Input: part model. Units: mm. Frame: model coordinates. A direction names the side the tool comes from. Round coordinates to 2 decimals unless told otherwise and drop trailing zeros. Loops run counter-clockwise (first coordinate to the right, second up) from the corner with the lowest first, then second, coordinate; pieces in that order, holes last. Notation, with made-up numbers: (0, -13) -> (35, -13) arc R25 ccw to (35, 14) -> close; hole circle Ø9 at (-5.5, 52). An arc over 180 degrees is marked (long way). Answer as a JSON object with one key per item and string values.
```python
from build123d import *

# Parameters (mm, degrees)
F0_W      = 12.7
F0_H      = 12.7
F1_DEPTH  = 76.2
F2_W      = 12.7
F2_H      = 25.4
F3_DEPTH  = 9.525
F4_W      = 12.7
F4_H      = 25.4
F5_DEPTH  = 9.525
F7_DEPTH  = 9.525
F9_DEPTH  = 9.525
F10_R     = 3.1496
F11_DEPTH = 25.4
F12_R     = 3.1496
F13_DEPTH = 25.4
F14_SIZE  = 2.54


with BuildPart() as f1:
    # F0 (on Top) → F1 (new body, symmetric)
    with BuildSketch(Plane.XY):
        Rectangle(F0_W, F0_H)
    extrude(amount=F1_DEPTH, both=True)

    # F2 (on face) → F3 (join)
    with BuildSketch(Plane(origin=(0, 6.35, 0), x_dir=(-1, 0, 0), z_dir=(0, 1, 0))):
        with Locations((0, -58.42)):
            Rectangle(F2_W, F2_H)
        with Locations((0, -12.7)):
            Rectangle(F2_W, F2_H)
        with Locations((0, 33.02)):
            Rectangle(F2_W, F2_H)
    extrude(amount=F3_DEPTH)

    # F4 (on face) → F5 (join)
    with BuildSketch(Plane.XZ.offset(6.35)):
        with Locations((0, 48.26)):
            Rectangle(F4_W, F4_H)
        with Locations((0, 2.54)):
            Rectangle(F4_W, F4_H)
        with Locations((0, -43.18)):
            Rectangle(F4_W, F4_H)
    extrude(amount=F5_DEPTH)

    # F6 (on face) → F7 (join)
    with BuildSketch(Plane(origin=(-6.35, 0, 0), x_dir=(0, -1, 0), z_dir=(-1, 0, 0))):
        Polygon((-6.35, 66.260369), (-6.35, 45.72), (-6.35, 44.788861), (6.35, 44.788861), (6.35, 60.96), (6.35, 66.260369), align=None)
        Polygon((-6.35, 20.32), (-6.35, 0), (6.35, 0), (6.35, 15.24), (6.35, 22.712743), (-6.35, 22.712743), align=None)
        Polygon((-6.35, -45.72), (-6.35, -50.8), (0, -50.8), (0, -19.05), (-6.35, -19.05), (-6.35, -25.4), align=None)
    extrude(amount=F7_DEPTH)

    # F8 (on face) → F9 (join)
    with BuildSketch(Plane.YZ.offset(6.35)):
        Polygon((6.35, -24.37056), (-6.35, -24.37056), (-6.35, -30.48), (-6.35, -49.77056), (6.35, -49.77056), (6.35, -45.72), (6.35, -25.4), align=None)
        Polygon((6.35, 35.56), (-6.35, 35.56), (-6.35, 15.24), (-6.35, 10.16), (6.35, 10.16), (6.35, 20.32), align=None)
        Polygon((6.35, 73.66), (-6.35, 73.66), (-6.35, 60.96), (-6.35, 48.26), (6.35, 48.26), align=None)
    extrude(amount=F9_DEPTH)

    # F10 (on face) → F11 (join)
    with BuildSketch(Plane.XY.offset(76.2)):
        Circle(F10_R)
    extrude(amount=F11_DEPTH)

    # F12 (on face) → F13 (join)
    with BuildSketch(Plane(origin=(0, 0, -76.2), x_dir=(1, 0, 0), z_dir=(0, 0, -1))):
        Circle(F12_R)
    extrude(amount=F13_DEPTH)

    # F14
    f14_edges = [f1.edges().sort_by_distance(p)[0] for p in [
        (15.875, -6.35, 60.96),
        (15.875, 6.35, 60.96),
        (6.35, -15.875, 48.26),
        (-6.35, -15.875, 48.26),
        (-15.875, -6.35, 55.524615),
        (-15.875, 6.35, 55.524615),
        (-6.35, 15.875, 33.02),
        (6.35, 15.875, 33.02),
        (15.875, 6.35, 22.86),
        (15.875, -6.35, 22.86),
        (6.35, -15.875, 2.54),
        (-6.35, -15.875, 2.54),
        (-15.875, -6.35, 11.356371),
        (-15.875, 6.35, 11.356371),
        (-6.35, 15.875, -12.7),
        (6.35, 15.875, -12.7),
        (-15.875, 6.35, -34.925),
        (-15.875, 0, -34.925),
        (-6.35, -15.875, -43.18),
        (6.35, -15.875, -43.18),
        (6.35, -6.35, -40.12528),
        (15.875, 6.35, -37.07056),
        (15.875, -6.35, -37.07056),
        (6.35, 15.875, -58.42),
        (-6.35, 15.875, -58.42),
    ]]
    chamfer(f14_edges, length=F14_SIZE)


solid = f1.part
```
1) Contact query for flat-ended pins moving along their axis: P1, Ø4, axis at x = -6.5, y = -11, coming from the -Z side; P2, Ø12, axis at x = -12, y = -2.5, coming from the +Z side; P3, Ø1.5, axis at x = 3, z = -37.5, coming from the +Y side. Output: stop coordinate, or through.
Output:
{"P1": "stops at z = -55.88", "P2": "stops at z = 76.2", "P3": "stops at y = 6.35"}
2) Section D-D, the plane z = -33. Output: boundary loops of the cut face in (x, y) (3 decimals).
Output:
{"outline": "(-15.875, 2.54) -> (-13.335, 0) -> (-6.35, 0) -> (-6.35, -13.335) -> (-3.81, -15.875) -> (3.81, -15.875) -> (6.35, -13.335) -> (6.35, -8.89) -> (8.89, -6.35) -> (13.335, -6.35) -> (15.875, -3.81) -> (15.875, 3.81) -> (13.335, 6.35) -> (-13.335, 6.35) -> (-15.875, 3.81) -> close"}
3) Section A-A, the plane y = 11.5. Output: boundary loops of the cut face in (x, z), plus the area to 3 significant figures.
Output:
{"outline": "(-6.35, -71.12) -> (6.35, -71.12) -> (6.35, -45.72) -> (-6.35, -45.72) -> close; (-6.35, -25.4) -> (6.35, -25.4) -> (6.35, 0) -> (-6.35, 0) -> close; (-6.35, 20.32) -> (6.35, 20.32) -> (6.35, 45.72) -> (-6.35, 45.72) -> close", "area": "968 mm^2"}
4) Section B-B, the plane x = -10.5. Output: boundary loops of the cut face in (y, z), plus the area to 3 significant figures.
Output:
{"outline": "(-6.35, 0) -> (6.35, 0) -> (6.35, 22.71) -> (-6.35, 22.71) -> close; (-6.35, 44.79) -> (6.35, 44.79) -> (6.35, 66.26) -> (-6.35, 66.26) -> close; (0, -50.8) -> (6.35, -50.8) -> (6.35, -19.05) -> (0, -19.05) -> close", "area": "763 mm^2"}
5) Section C-C, the plane z = 13.5. Output: boundary loops of the cut face in (x, y) (3 decimals).
Output:
{"outline": "(-15.875, -3.81) -> (-13.335, -6.35) -> (-6.35, -6.35) -> (-6.35, -13.335) -> (-3.81, -15.875) -> (3.81, -15.875) -> (6.35, -13.335) -> (6.35, -6.35) -> (13.335, -6.35) -> (15.875, -3.81) -> (15.875, 3.81) -> (13.335, 6.35) -> (-13.335, 6.35) -> (-15.875, 3.81) -> close"}
6) Draft query along Z for faces 1 (the face through (11, 0, -49.771)), 2 (the face through (0, 11, -45.72)), 3 (the face through (0, -6.35, 64)). Return one class per face: +Z half, -Z half, draft (parallel to the pull), parting line (faces both ways), or undercut.
Output:
{"face 1": "-Z half", "face 2": "undercut", "face 3": "draft"}
7) Ray query, probe 1 along Z at (x, y) = (-4.5, -11.5); probe 2 along Z at (x, y) = (-12.5, -2); probe 3 along X at (y, z) = (6, -57.5). Return the intervals inside material, ascending.
Output:
{"probe 1": "z = -55.88 to -30.48, -10.16 to 15.24, 35.56 to 60.96", "probe 2": "z = 0 to 22.71, 44.79 to 66.26", "probe 3": "x = -6.35 to 6.35"}
8) Reachability of faces 4 (the face through (0, -11, 60.96)), 5 (the face through (0, -11, 15.24)), 6 (the face through (-11, 0, 66.26)), 7 (the face through (11, 0, 10.16)) from +Z, -Z, +X, -X, +Y, -Y: full face, straight path, thin tool, end or side. Return the list, or none.
Output:
{"face 4": "+Z, +X, -X, -Y", "face 5": "+X, -X, -Y", "face 6": "+Z, -X, +Y, -Y", "face 7": "+X, +Y, -Y"}
